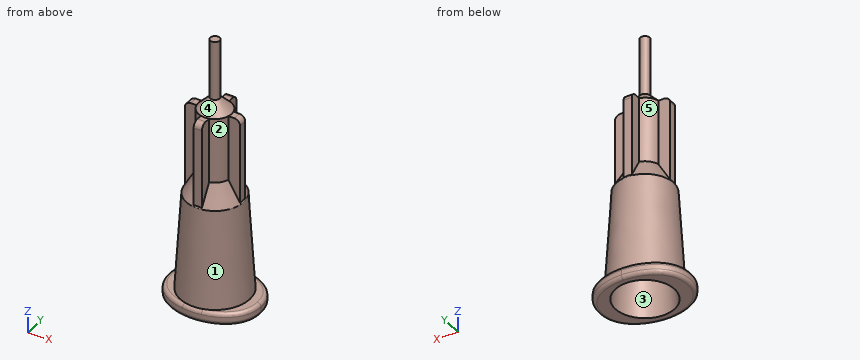
```python
from build123d import *

# Parameters (mm, degrees)
BOSS_EXTRUDE1_DEPTH = 0.35
CIRPATTERN1_COUNT   = 4
SKETCH4_R           = 5.5
CUT_EXTRUDE2_DEPTH  = 18.397413601
FILLET1_R           = 0.3
SKETCH6_W           = 0.4
SKETCH6_H           = 5
FILLET2_R           = 0.5


with BuildPart() as part:
    # Sketch1 → Revolve1 (revolve)
    with BuildSketch(Plane(origin=(0, 0, 0), x_dir=(1, 0, 0), z_dir=(0, 1, 0))):
        Polygon((2.5, 0), (3, 0), (3.9, 0), (3.9, -1), (2.938475611, -1), (2.424366542, -9.225745104), (1.4, -11), (1.4, -16.5), (0.4, -16.5), (0.4, -8), (2, -8), align=None)
    revolve(axis=Axis((0, 0, 16.5), (0, 0, -1)))

    # Sketch2 → Boss-Extrude1 (add, symmetric)
    with BuildSketch(Plane(origin=(0, 0, 0), x_dir=(1, 0, 0), z_dir=(0, 1, 0))):
        Polygon((2.35, -9.094744112), (1.25, -11), (1.25, -16.5), (2.35, -16.5), align=None)
    boss_extrude1 = extrude(amount=BOSS_EXTRUDE1_DEPTH, both=True)

    # CirPattern1: Boss-Extrude1 ×4 about axis
    cirpattern1_axis = Axis((0, 0, 0), (0, 0, 1))
    for i in range(1, CIRPATTERN1_COUNT):
        add(boss_extrude1.rotate(cirpattern1_axis, i * 360 / CIRPATTERN1_COUNT))

    # Sketch4 → Cut-Extrude2 (cut, through all)
    with BuildSketch(Plane(origin=(0, 0, 0), x_dir=(-1, 0, 0), z_dir=(0, 0, -1))):
        Circle(SKETCH4_R)
        with BuildLine():
            add(Edge.make_bspline(
                [(0, 3.2), (-1.681599767, 3.2), (-3.9, 2.322621385), (-3.9, 0)],
                knots=[0, 0, 0, 0, 1, 1, 1, 1], degree=3))
            add(Edge.make_bspline(
                [(0, -3.2), (-1.681599767, -3.2), (-3.9, -2.322621385), (-3.9, 0)],
                knots=[0, 0, 0, 0, 1, 1, 1, 1], degree=3))
            add(Edge.make_bspline(
                [(0, -3.2), (1.681599767, -3.2), (3.9, -2.322621385), (3.9, 0)],
                knots=[0, 0, 0, 0, 1, 1, 1, 1], degree=3))
            add(Edge.make_bspline(
                [(0, 3.2), (1.681599767, 3.2), (3.9, 2.322621385), (3.9, 0)],
                knots=[0, 0, 0, 0, 1, 1, 1, 1], degree=3))
        make_face(mode=Mode.SUBTRACT)
    extrude(amount=-CUT_EXTRUDE2_DEPTH, mode=Mode.SUBTRACT)

    # Fillet1
    fillet1_edges = [part.edges().sort_by_distance(p)[0] for p in [
        (2.666281983, -2.412027807, 0),
        (-2.666281983, -2.412027807, 0),
        (-2.666281983, 2.412027807, 0),
        (2.666281983, 2.412027807, 0),
        (2.666282105, -2.412027711, 1),
        (-2.666282105, -2.412027711, 1),
        (-2.666282105, 2.412027711, 1),
        (2.666282105, 2.412027711, 1),
    ]]
    fillet(fillet1_edges, radius=FILLET1_R)

    # Sketch5 → Revolve2 (revolve)
    with BuildSketch(Plane(origin=(0, 0, 0), x_dir=(1, 0, 0), z_dir=(0, 1, 0)), mode=Mode.PRIVATE) as revolve2_sk:
        Polygon((0, -16.5), (1.4, -16.5), (0.4, -17.5), (0, -17.5), align=None)
    revolve(revolve2_sk.sketch.rotate(Axis((0, 0, 0), (0, 0, 1)), 171.528954844), axis=Axis((0, 0, 0), (0, 0, 1)))

    # Sketch6 → Revolve3 (revolve)
    with BuildSketch(Plane(origin=(0, 0, 0), x_dir=(1, 0, 0), z_dir=(0, 1, 0)), mode=Mode.PRIVATE) as revolve3_sk:
        with Locations((0.2, -20)):
            Rectangle(SKETCH6_W, SKETCH6_H)
    revolve(revolve3_sk.sketch.rotate(Axis((0, 0, 22.5), (0, 0, -1)), 188.471045156), axis=Axis((0, 0, 22.5), (0, 0, -1)))

    # Fillet2
    fillet2_edges = [part.edges().sort_by_distance(p)[0] for p in [
        (2.35, 0, 16.5),
        (0, 2.35, 16.5),
        (-2.35, 0, 16.5),
        (0, -2.35, 16.5),
    ]]
    fillet(fillet2_edges, radius=FILLET2_R)


solid = part.part
```
CAD build for the part. Positions are in the model's coordinates, mm. Face numbers are marked on the shaded views. A direction names the side the tool comes from. Coordinates: 2 decimals unless noted, no trailing zeros. Write each loop counter-clockwise with the first axis right and the second up, starting at its lowest first coordinate (ties: lowest second). Pieces come first, ordered by that corner, then holes.
(1) Cut at A-A, the plane z = 14.75. List the corners of the cut face in (x, y).
(2) Flat gauge pins, fed straight in: pin 1 (0.5 mm diameter, centred on x = 1.5, y = 0, fed in from +Z); pin 2 (2.5 mm diameter, centred on x = -2, y = -0.5, fed in from +Z); pin 3 (2 mm diameter, centred on x = 1, z = 13, fed in from +Y). Where does each tip first touch, or does it go through?
(3) 3-axis set-ups, long thin cutter, end or side, ignore diameter. For the marked faces 4 and 5: which of +Z, -Z, +X, -X, +Y, -Y reach the whole face in a straight line?
(4) Two-plate mould, pull along X, no slides. Class the marked faces 1, 2 and 3: +X half, -X half, draft (parallel to the pull), parting line (faces both ways), or undercut.
(5) Drill centre lines: probe 1 along Y at (x, z) = (0, 10.75); probe 2 along Z at (x, y) = (3, 1.5); probe 3 along Z at (x, y) = (0, 0). Where is each one in solid material? Low to high.
Geometry says:
1. outline: (-2.35, -0.35) - (-1.36, -0.35) arc R1.4 ccw to (-0.35, -1.36) - (-0.35, -2.35) - (0.35, -2.35) - (0.35, -1.36) arc R1.4 ccw to (1.36, -0.35) - (2.35, -0.35) - (2.35, 0.35) - (1.36, 0.35) arc R1.4 ccw to (0.35, 1.36) - (0.35, 2.35) - (-0.35, 2.35) - (-0.35, 1.36) arc R1.4 ccw to (-1.36, 0.35) - (-2.35, 0.35) - close; hole circle Ø0.8 at (0, 0)
2. pin 1: stops at z = 16.65
2. pin 2: stops at z = 17.09
2. pin 3: stops at y = 2.35
3. face 4: +Z
3. face 5: +Z, -X, +Y
4. face 1: parting line
4. face 2: +X half
4. face 3: undercut
5. probe 1: y = -2.35 to -0.4, 0.4 to 2.35
5. probe 2: z = 0 to 1
5. probe 3: z = 16.5 to 22.5
